Work out the finished part from the listing and answer in its coordinate system (mm). Face numbers are marked on the shaded views. A direction names the side the tool comes from. Round coordinates to 2 decimals unless told otherwise and drop trailing zeros. Order: outer loops, then holes, each group sorted by start corner. A loop starts at its lowest first (then second) coordinate and runs counter-clockwise, first axis right, second up. Notation, with made-up numbers: (37.5, 26) - (63.5, 26) arc R28 cw to (63.5, 58) - close; hole circle Ø8 at (55, 71). An arc over 180 degrees is marked (long way). Answer in a Markdown table with one row per item.
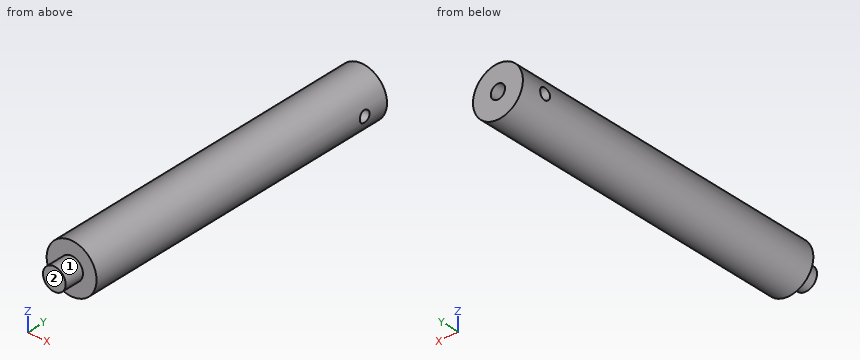
from build123d import *

# Parameters (mm, degrees)
F0_R     = 8.8011
F1_DEPTH = 124.46
F2_R     = 8.8011
F2_R_2   = 4
F3_DEPTH = 7
F4_R     = 2.5
F5_DEPTH = 18
F8_R     = 1.984375
F9_DEPTH = 17.6032


with BuildPart() as f1:
    # F0 (on Front) → F1 (new body)
    with BuildSketch(Plane.XZ):
        Circle(F0_R)
    extrude(amount=F1_DEPTH)

    # F2 (on face) → F3 (cut)
    with BuildSketch(Plane.XZ.offset(124.46)):
        Circle(F2_R)
        Circle(F2_R_2, mode=Mode.SUBTRACT)
    extrude(amount=-F3_DEPTH, mode=Mode.SUBTRACT)

    # F4 (on face) → F5 (cut)
    with BuildSketch(Plane(origin=(0, 0, 0), x_dir=(-1, 0, 0), z_dir=(0, 1, 0))):
        Circle(F4_R)
    extrude(amount=-F5_DEPTH, mode=Mode.SUBTRACT)

    # F8 (on face) → F9 (cut, through all)
    with BuildSketch(Plane(origin=(-8.8011, 0, 0), x_dir=(0, -1, 0), z_dir=(-1, 0, 0))):
        with Locations((9, 0)):
            Circle(F8_R)
    extrude(amount=-F9_DEPTH, mode=Mode.SUBTRACT)


solid = f1.part
1) Find section A-A, the plane z = 0. Give the vertices of the cut face in (x, y).
Filled in:
| item | result |
|---|---|
| outline | (-8.8, -117.46) - (-4, -117.46) - (-4, -124.46) - (4, -124.46) - (4, -117.46) - (8.8, -117.46) - (8.8, -10.98) - (2.5, -10.98) - (2.5, -18) - (-2.5, -18) - (-2.5, -10.98) - (-8.8, -10.98) - close; (-8.8, -7.02) - (-2.5, -7.02) - (-2.5, 0) - (-8.8, 0) - close; (2.5, -7.02) - (8.8, -7.02) - (8.8, 0) - (2.5, 0) - close |
2) Each of these flat-tipped pins is pushed along its axis until it touches: pin 1 (4 mm diameter, centred on x = 0, z = 0, fed in from +Y); pin 2 (4 mm diameter, centred on x = 5, y = -108, fed in from +Z); pin 3 (5 mm diameter, centred on y = -13.5, z = -1, fed in from +X); pin 4 (6 mm diameter, centred on x = -6.5, z = 5, fed in from -Y). Where does it stop, or does it pass through?
Filled in:
| item | result |
|---|---|
| pin 1 | stops at y = -18 |
| pin 2 | stops at z = 8.27 |
| pin 3 | stops at x = 8.8 |
| pin 4 | stops at y = -117.46 |
3) Find section D-D, the plane x = 6.75. Give the vertices of the cut face in (y, z), then the cut area to 3 significant figures.
Filled in:
| item | result |
|---|---|
| outline | (-117.46, -5.65) - (0, -5.65) - (0, 5.65) - (-117.46, 5.65) - close; hole circle Ø3.97 at (-9, 0) |
| area | 1,310 mm^2 |
4) Find the intervals of material crossed by probe 1 along X at (y, z) = (-6.5, 0); probe 2 along Y at (x, z) = (-5.25, 0.25), in increasing order. Write a range as from..to.
Filled in:
| item | result |
|---|---|
| probe 1 | x = -8.8..-2.5, 2.5..8.8 |
| probe 2 | y = -117.46..-10.97, -7.03..0 |
5) Which of the six approach directions +Z, -Z, +X, -X, +Y, -Y give full straight-line access (tool end or side, diameter ignored) to the marked faces 1 and 2?
Filled in:
| item | result |
|---|---|
| face 1 | -Y |
| face 2 | +Z, -Z, +X, -X, -Y |
6) Find section C-C, the plane x = 0. Give the vertices of the cut face in (y, z).
Filled in:
| item | result |
|---|---|
| outline | (-124.46, -4) - (-117.46, -4) - (-117.46, -8.8) - (0, -8.8) - (0, -2.5) - (-18, -2.5) - (-18, 2.5) - (0, 2.5) - (0, 8.8) - (-117.46, 8.8) - (-117.46, 4) - (-124.46, 4) - close |
7) Find section B-B, the plane y = -9.5. Give the vertices of the cut face in (x, z).
Filled in:
| item | result |
|---|---|
| outline | (-8.59, -1.92) arc R8.8 ccw to (8.59, -1.92) - (1.6, -1.92) arc R2.5 cw to (-1.6, -1.92) - close; (-8.59, 1.92) - (-1.6, 1.92) arc R2.5 cw to (1.6, 1.92) - (8.59, 1.92) arc R8.8 ccw to start |
